Read the model definition and answer for the solid it produces. Units are mm, in the model's axes. Round coordinates to 2 decimals unless told otherwise and drop trailing zeros. Write each loop counter-clockwise with the first axis right and the second up, starting at its lowest first coordinate (ties: lowest second). Pieces come first, ordered by that corner, then holes.
from build123d import *

# Parameters (mm, degrees)
F1_DEPTH       = 7.9375
F2_D           = 8.4328
F2_CSINK_D     = 16.6624
F2_CSINK_ANGLE = 82


with BuildPart() as f1:
    # F0 (on Front) → F1 (new body)
    with BuildSketch(Plane.XZ):
        with BuildLine():
            Line((38.1, -63.5), (38.1, 0))
            ThreePointArc((38.1, 0), (0, 38.1), (-38.1, 0))
            Line((-38.1, 0), (-38.1, -63.5))
            Line((-38.1, -63.5), (38.1, -63.5))
        make_face()
    extrude(amount=F1_DEPTH)

    # F2 (through all)
    with Locations(Plane(origin=(0, 0, 0), x_dir=(1, 0, 0), z_dir=(0, 1, 0))):
        with Locations((-25.4, 44.45), (25.4, 44.45)):
            CounterSinkHole(F2_D / 2, F2_CSINK_D / 2, counter_sink_angle=F2_CSINK_ANGLE)


solid = f1.part
Q1. Flat-ended cylindrical pins translate along their axes: pin 1 Ø5 at (x, z) = (-25.4, -44.45) entering from +Y; pin 2 Ø4 at (x, y) = (22.5, -1) entering from +Z; pin 3 Ø13.5 at (x, z) = (25.4, -44.45) entering from +Y; pin 4 Ø4 at (x, y) = (-15.5, -1) entering from +Z. Find the tip coordinate at first contact, or state that the pin passes through.
Verdict:
pin 1: passes through
pin 2: stops at z = 32.11
pin 3: stops at y = -1.82
pin 4: stops at z = 35.63
Q2. Section B-B (x = 25.4) is taken. Determine the outline of the cut face in (y, z).
Verdict:
outline: (-7.94, -63.5) - (0, -63.5) - (0, -52.78) - (-4.73, -48.67) - (-7.94, -48.67) - close; (-7.94, -40.23) - (-4.73, -40.23) - (0, -36.12) - (0, 28.4) - (-7.94, 28.4) - close
Q3. Section D-D (z = 25) is taken. Determine the outline of the cut face in (x, y).
Verdict:
outline: (-28.75, -7.94) - (28.75, -7.94) - (28.75, 0) - (-28.75, 0) - close
Q4. Section A-A (z = -44.45) is taken. Determine the outline of the cut face in (x, y), then the cut area to 3 significant figures.
Verdict:
outline: (-38.1, -7.94) - (-29.62, -7.94) - (-29.62, -4.73) - (-33.73, 0) - (-38.1, 0) - close; (-21.18, -7.94) - (21.18, -7.94) - (21.18, -4.73) - (17.07, 0) - (-17.07, 0) - (-21.18, -4.73) - close; (29.62, -7.94) - (38.1, -7.94) - (38.1, 0) - (33.73, 0) - (29.62, -4.73) - close
area: 432 mm2
Q5. Straight lines are drawn through the part: probe 1 along X at (y, z) = (-7.05, -44.45); probe 2 along X at (y, z) = (-2.75, -43.5); probe 3 along Z at (x, y) = (27.5, -1.25). For each, find the intervals that lie inside material, in ascending order.
Verdict:
probe 1: x = -38.1 to -29.62, -21.18 to 21.18, 29.62 to 38.1
probe 2: x = -38.1 to -31.26, -19.54 to 19.54, 31.26 to 38.1
probe 3: z = -63.5 to -51.38, -37.52 to 26.37
Q6. Determine the mould class of faces 1 (the flat face through (38.1, -4, -32)), 2 (the conical face through (-20.988, -4.504, -44.644)), 3 (the conical face through (29.812, -4.504, -44.644)), 4 (the flat face through (-1, -4, -63.5)) for opening direction X: pulls with the +X half, pulls with the -X half, needs draft (parallel to the pull), parting line crosses it, or undercut.
Verdict:
face 1: pulls with the +X half
face 2: undercut
face 3: undercut
face 4: needs draft
Q7. Section C-C (y = -6.75) is taken. Determine the outline of the cut face in (x, z).
Verdict:
outline: (-38.1, -63.5) - (38.1, -63.5) - (38.1, 0) arc R38.1 ccw to (-38.1, 0) - close; hole circle Ø8.43 at (-25.4, -44.45); hole circle Ø8.43 at (25.4, -44.45)
